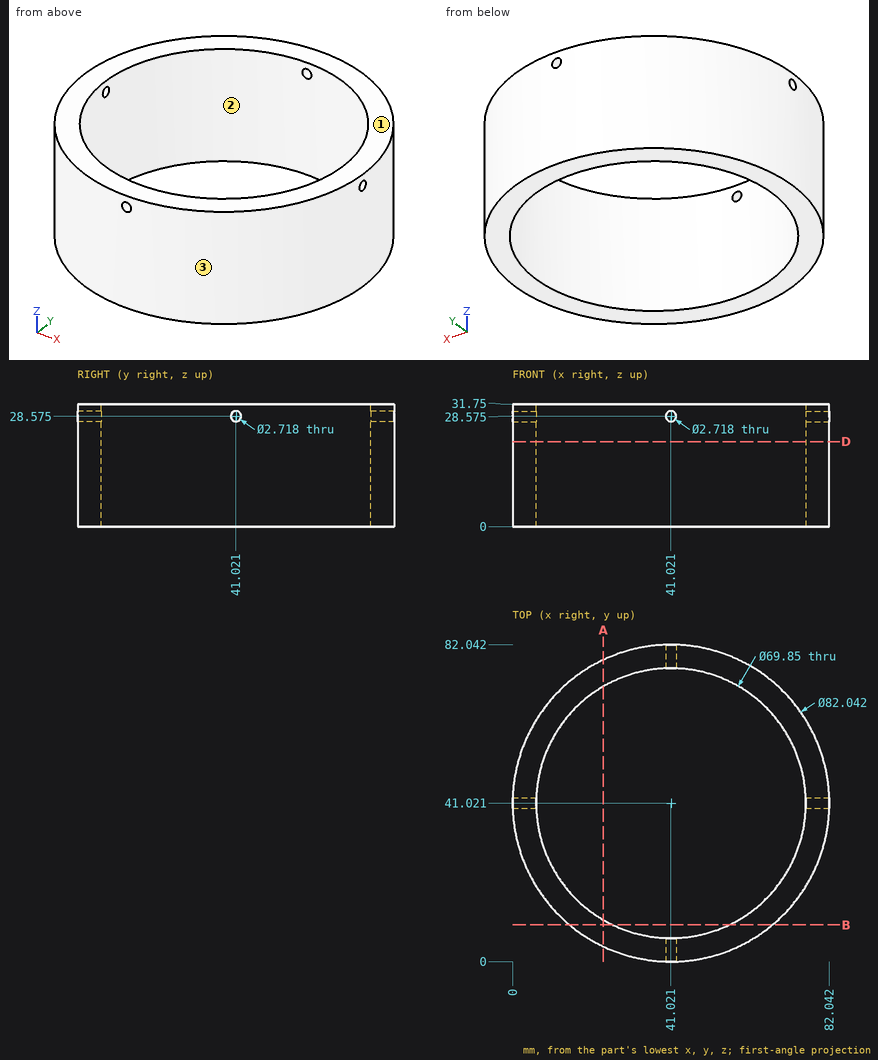
Source: three-view drawing plus pictorial views. Frame: mm from the lowest corner of the part. Coordinates: 2 decimals unless noted, no trailing zeros. Order: outer loops, then holes, each group sorted by start corner. A loop starts at its lowest first (then second) coordinate and runs counter-clockwise, first axis right, second up.
Item 1: Material intervals for line 1 (Y direction, x = 39.5, z = 3.5); line 2 (Y direction, x = 47, z = 28); line 3 (X direction, y = 67, z = 29) (1 decimal), sorted ascending.
Output values:
line 1: y = 0.03 to 6.13, 75.91 to 82.01
line 2: y = 0.44 to 6.61, 75.43 to 81.6
line 3: x = 9.3 to 17.7, 64.4 to 72.8
Item 2: Pull-direction query (Y, two-part tool) for the marked faces 1, 2 and 3; classes: pulls with the +Y half, pulls with the -Y half, needs draft (parallel to the pull), parting line crosses it, or undercut.
Output values:
face 1: needs draft
face 2: undercut
face 3: parting line crosses it
Item 3: Cut plane B-B (y = 9.5). Return loops of the section in (x, z).
Output values:
outline: (14.77, 0) - (25.98, 0) - (25.98, 31.75) - (14.77, 31.75) - close; (56.06, 0) - (67.27, 0) - (67.27, 31.75) - (56.06, 31.75) - close
Item 4: First-contact query: P1, Ø3, axis at y = 41.021, z = 28.575, coming from the +X side; P2, Ø1.5, axis at y = 73.5, z = 23.5, coming from the -X side; P3, Ø2, axis at x = 44.5, z = 21, coming from the +Y side; P4, Ø1, axis at y = 34.5, z = 11.5, coming from the +X side. Flat tips, straight axial feed; report the tip coordinate or a pass-through.
Output values:
P1: stops at x = 82.04
P2: stops at x = 15.02
P3: stops at y = 81.97
P4: stops at x = 81.6
Item 5: Cut plane A-A (x = 23.5). Return loops of the section in (y, z), plus the area to 3 significant figures.
Output values:
outline: (3.93, 0) - (10.81, 0) - (10.81, 31.75) - (3.93, 31.75) - close; (71.23, 0) - (78.11, 0) - (78.11, 31.75) - (71.23, 31.75) - close
area: 437 mm2
Item 6: Cut plane D-D (z = 22). Return loops of the section in (x, y) (3 decimals).
Output values:
outline: circle Ø82.042 at (41.021, 41.021); hole circle Ø69.85 at (41.021, 41.021)
